Could you check a few things on this drawing? It's one solid part, dimensions in mm from its lowest x, y, z. A direction names the side the tool comes from. Round coordinates to 2 decimals unless told otherwise and drop trailing zeros. Loops run counter-clockwise (first coordinate to the right, second up) from the corner with the lowest first, then second, coordinate; pieces in that order, holes last. Notation, with made-up numbers: (-5, 5.25) -> (25, 5.25) arc R21 cw to (25, 22.25) -> close; hole circle Ø6 at (21, -40). An arc over 180 degrees is marked (long way). Use one line per item in the form item = value. Start each with the question number.
Item 1: Thinking about a two-plate mould opening in X: for the marked faces 1, 2 and 3, which applies, released by +X, released by -X, zero draft, split by the parting line, or undercut?
Item 2: If we section it at B-B (y = 61): Write out the boundary of the cut face in (x, z), then the cut area to 3 significant figures.
Item 3: If I drill on L1, parallel to X at y = 17, z = 10.5; L2, parallel to X at y = 88, z = 8.5; L3, parallel to X at y = 80.75, z = 10 (3 decimals), over which ranges is the centre line in solid material (lowest first)? Write a range as [from, to].
Item 4: If we section it at A-A (x = 312): Write out the boundary of the cut face in (y, z).
Item 5: I'm going to push flat-ended pins straight in: pin 1 Ø6 at (x, z) = (322, 12.5) entering from -Y; pin 2 Ø2.5 at (y, z) = (10, 10) entering from -X. Where does each tip first touch, or does it pass through?
Item 6: For the marked faces 4 and 5, which set-ups out of +Z, -Z, +X, -X, +Y, -Y let a thin tool reach every point of the face, with its end or its side?
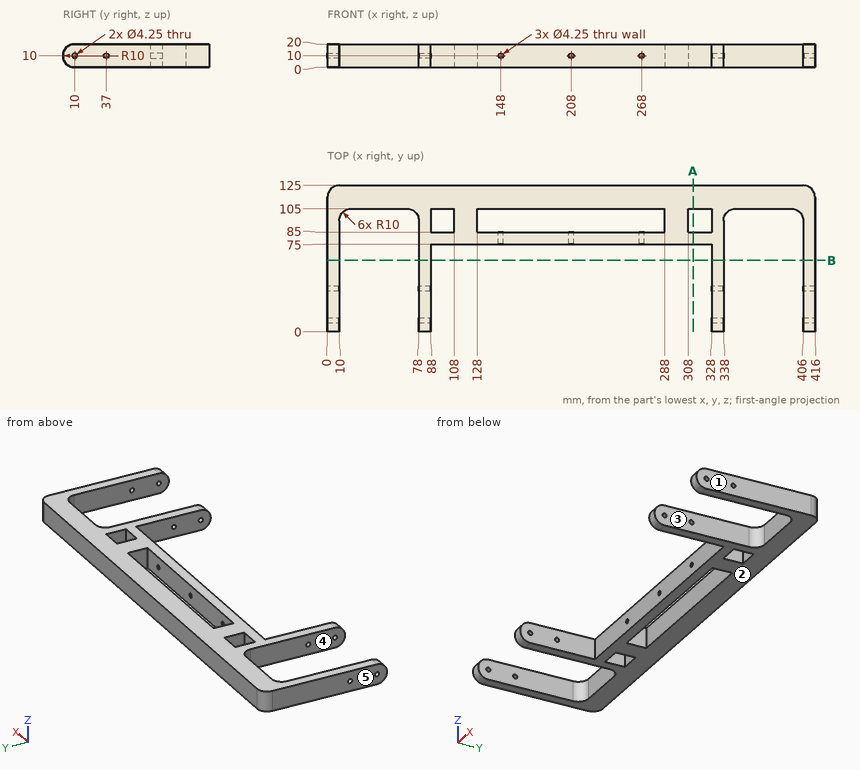
Values found:
q1.face_1 = released by +X
q1.face_2 = zero draft
q1.face_3 = undercut
q2.outline = (0, 0) -> (10, 0) -> (10, 20) -> (0, 20) -> close; (78, 0) -> (88, 0) -> (88, 20) -> (78, 20) -> close; (328, 0) -> (338, 0) -> (338, 20) -> (328, 20) -> close; (406, 0) -> (416, 0) -> (416, 20) -> (406, 20) -> close
q2.area = 800 mm2
q3.L1 = [0, 10], [78, 88], [328, 338], [406, 416]
q3.L2 = [0, 10], [78, 88], [108, 128], [288, 308], [328, 338], [406, 416]
q3.L3 = [0, 10], [78, 145.875], [150.125, 205.875], [210.125, 265.875], [270.125, 338], [406, 416]
q4.outline = (75, 0) -> (85, 0) -> (85, 20) -> (75, 20) -> close; (105, 0) -> (125, 0) -> (125, 20) -> (105, 20) -> close
q5.pin_1 = 75
q5.pin_2 = through
q6.face_4 = +Z, -Z, -Y
q6.face_5 = +Z, -Z, -X, +Y, -Y
